Autodesk Inventor part; units mm, degrees
ref_plane "YZ Plane" through (0, 0, 0) normal (1, 0, 0) x (0, 1, 0)
ref_plane "XZ Plane" through (0, 0, 0) normal (0, 1, 0) x (-1, 0, 0)
ref_plane "XY Plane" through (0, 0, 0) normal (0, 0, 1) x (1, 0, 0)
sketch "Boceto1" plane through (0, 0, 0) normal (0, 1, 0) x (-1, 0, 0)
  line L0 (0, 0) -> (240, 0)
  line L1 (240, 0) -> (240, -25)
  line L2 (240, -25) -> (0, -25)
  line L3 (0, -25) -> (0, 0)
  dimension "d0" = 240
  dimension "d1" = 25
extrude "Extrusión1" add sketch "Boceto1" along normal blind 58
sketch "Boceto2" plane through (0, 58, 0) normal (0, 1, 0) x (1, 0, 0)
  line L0 (0, 25) -> (-240, 25)
  line L1 (-240, 25) -> (-240, 0)
  line L2 (-240, 0) -> (0, 0)
  line L3 (0, 0) -> (0, 25)
  line L4 (-213, 2.5) -> (-193, 2.5)
  line L5 (-193, 2.5) -> (-193, 22.5)
  line L6 (-193, 22.5) -> (-213, 22.5)
  line L7 (-213, 22.5) -> (-213, 2.5)
  line L8 (-213, 2.5) -> (-193, 22.5) construction
  line L9 (-193, 2.5) -> (-213, 22.5) construction
  line L10 (-27, 22.5) -> (-47, 22.5)
  line L11 (-47, 22.5) -> (-47, 2.5)
  line L12 (-47, 2.5) -> (-27, 2.5)
  line L13 (-27, 2.5) -> (-27, 22.5)
  line L14 (-27, 22.5) -> (-47, 2.5) construction
  line L15 (-47, 22.5) -> (-27, 2.5) construction
  point P0 (-203, 12.5)
  point P1 (-37, 12.5)
  dimension "d10" = 20
  dimension "d11" = 20
  dimension "d12" = 20
  dimension "d13" = 20
  dimension "d14" = 27
  dimension "d15" = 146
extrude "Extrusión2" cut sketch "Boceto2" against normal blind 58 contours L7 L6 L5 L4 | L13 L12 L11 L10
sketch "Boceto3" plane through (0, 0, 0) normal (1, 0, 0) x (0, 0, -1)
  line L0 (0, 0) -> (25, 0)
  line L1 (25, 0) -> (25, 58)
  line L2 (0, 58) -> (25, 58)
  line L3 (0, 0) -> (0, 58)
  line L4 (0, 0) -> (0, 58)
  line L5 (1.7, 52.5054) -> (1.7, 56.3)
  line L6 (1.7, 56.3) -> (23.3, 56.3)
  line L7 (25, 0) -> (25, 58)
  line L8 (22.5, 0) -> (2.5, 0)
  line L9 (7.4249, 0) -> (7.4249, 1.7)
  line L10 (7.4249, 1.7) -> (1.7, 1.7)
  line L11 (1.7, 52.5054) -> (1.7, 1.7)
  line L12 (7.4249, 1.7) -> (23.3, 1.7)
  line L13 (23.3, 1.7) -> (23.3, 56.3)
  point P0 (12.9, 29.7431)
  point P1 (2.5, 58)
extrude "Extrusión3" cut sketch "Boceto3" against normal blind 240 contours L10 L11 L5 L6 L13 L12
properties part number "Travesaño"
CAD build for the part. Positions are in the model's coordinates, mm. A direction names the side the tool comes from. Give positions to 0.01 mm unless a question says otherwise; leave off trailing zeros. Order: outer loops, then holes, each group sorted by start corner. A loop starts at its lowest first (then second) coordinate and runs counter-clockwise, first axis right, second up.
(1) Saw through at B-B, the plane y = 25. Give the cut face in (x, z), then the cut area to 3 significant figures.
(2) Tool access for faces 5 (the flat face through (-118, 1.7, -12)), 6 (the flat face through (-118, 58, -12)): list every direction of +Z, -Z, +X, -X, +Y, -Y with a clear straight run to the whole face (end or side of a thin tool).
(3) Saw through at D-D, the plane x = -80.5. Give the cut face in (y, z), then the cut area to 3 significant figures.
(4) Mould opens along Z. For faces 1 (the flat face through (-118, 56.3, -12)), 2 (the flat face through (-118, 29, -1.7)), 3 (the flat face through (0, 27, -24)), 4 (the flat face through (-118, 29, 0)) say: released by +Z, released by -Z, zero draft, split by the parting line, or undercut.
(5) Saw through at C-C, the plane z = -20.5. Give the cut face in (x, y).
(6) Saw through at A-A, the plane x = -38. Give the cut face in (y, z), then the cut area to 3 significant figures.
(7) Drill centre lines: L1, parallel to Y at x = -170.5, z = -21.75; L2, parallel to Z at x = -120, y = 50. Where is each one in solid material? Low to high.
Results found:
1. outline: (-240, -25) - (0, -25) - (0, -23.3) - (-240, -23.3) - close; (-240, -1.7) - (0, -1.7) - (0, 0) - (-240, 0) - close
1. area: 816 mm2
2. face 5: +X, -X
2. face 6: +Z, -Z, +X, -X, +Y
3. outline: (0, -25) - (58, -25) - (58, 0) - (0, 0) - close; hole (1.7, -23.3) - (56.3, -23.3) - (56.3, -1.7) - (1.7, -1.7) - close
3. area: 271 mm2
4. face 1: undercut
4. face 2: undercut
4. face 3: zero draft
4. face 4: released by +Z
5. outline: (-240, 0) - (-213, 0) - (-213, 1.7) - (-240, 1.7) - close; (-240, 56.3) - (-213, 56.3) - (-213, 58) - (-240, 58) - close; (-193, 0) - (-47, 0) - (-47, 1.7) - (-193, 1.7) - close; (-193, 56.3) - (-47, 56.3) - (-47, 58) - (-193, 58) - close; (-27, 0) - (0, 0) - (0, 1.7) - (-27, 1.7) - close; (-27, 56.3) - (0, 56.3) - (0, 58) - (-27, 58) - close
6. outline: (0, -25) - (58, -25) - (58, -22.5) - (56.3, -22.5) - (56.3, -23.3) - (1.7, -23.3) - (1.7, -22.5) - (0, -22.5) - close; (0, -2.5) - (1.7, -2.5) - (1.7, -1.7) - (56.3, -1.7) - (56.3, -2.5) - (58, -2.5) - (58, 0) - (0, 0) - close
6. area: 203 mm2
7. L1: y = 0 to 1.7, 56.3 to 58
7. L2: z = -25 to -23.3, -1.7 to 0
